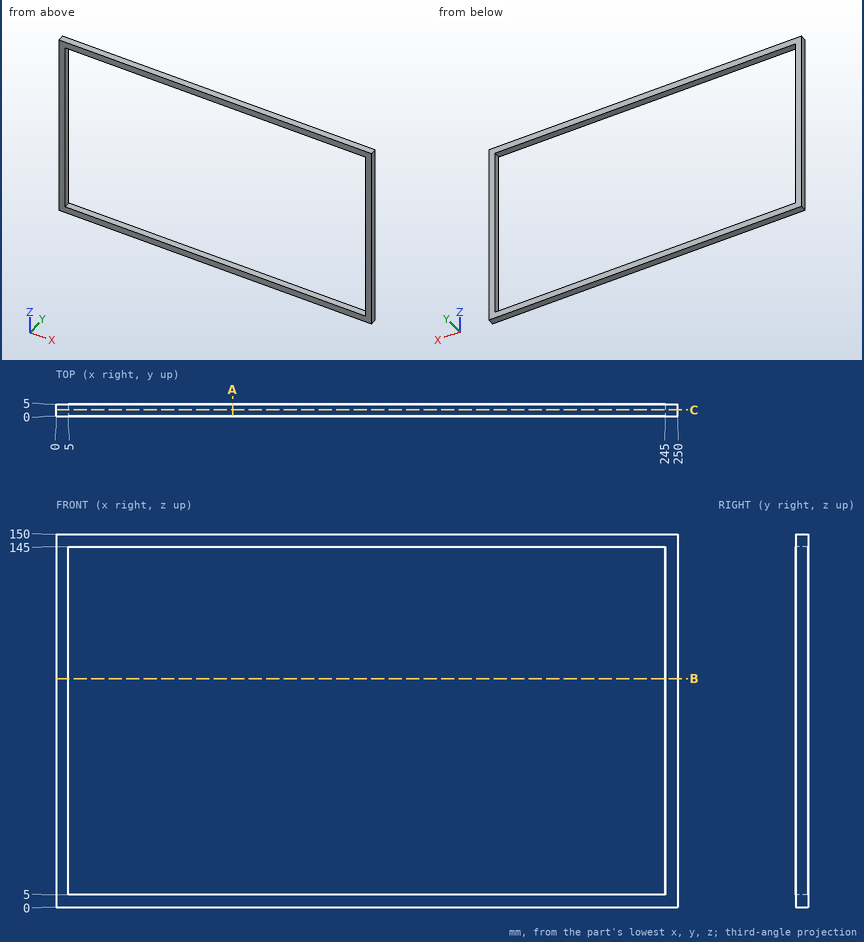
Print and shaded views of the part. All mm, measured from the part's lowest x, y and z. Give positions to 0.01 mm unless a question says otherwise; leave off trailing zeros. Loops run counter-clockwise (first coordinate to the right, second up) from the corner with the lowest first, then second, coordinate; pieces in that order, holes last. Notation, with made-up numbers: (23.25, 69) -> (74.25, 69) arc R6 ccw to (74.25, 78) -> close; hole circle Ø4 at (-40, 55). An arc over 180 degrees is marked (long way). Use a Markdown table: item, result.
1. Slice it at C-C (y = 2.6). List the corners of the cut face in (x, z).
Check result:
| item | result |
|---|---|
| outline | (0, 0) -> (250, 0) -> (250, 150) -> (0, 150) -> close; hole (5, 5) -> (245, 5) -> (245, 145) -> (5, 145) -> close |
2. Wall check: L1, parallel to Z at x = 47.5, y = 1.5; L2, parallel to X at y = 3.4, z = 139. Give the ranges that are in metal, low to high. Write a range as [from, to].
Check result:
| item | result |
|---|---|
| L1 | z = [0, 5], [145, 150] |
| L2 | x = [0, 5], [245, 250] |
3. Flat gauge pin, fed straight in: pin 1 (2.5 mm diameter, centred on y = 1.5, z = 109, fed in from -X). Where does the tip first touch, or does it go through?
Check result:
| item | result |
|---|---|
| pin 1 | stops at x = 0 |
4. Slice it at B-B (z = 92). List the corners of the cut face in (x, y).
Check result:
| item | result |
|---|---|
| outline | (0, 0) -> (5, 0) -> (5, 5) -> (0, 5) -> close; (245, 0) -> (250, 0) -> (250, 5) -> (245, 5) -> close |
5. Slice it at A-A (x = 71). List the corners of the cut face in (y, z), plus the area to 3 significant figures.
Check result:
| item | result |
|---|---|
| outline | (0, 0) -> (5, 0) -> (5, 5) -> (0, 5) -> close; (0, 145) -> (5, 145) -> (5, 150) -> (0, 150) -> close |
| area | 50.0 mm^2 |
